Here's how the part is built. I have some questions about the finished solid (model axes, mm). A direction names the side the tool comes from. Round coordinates to 2 decimals unless told otherwise and drop trailing zeros. Loops run counter-clockwise (first coordinate to the right, second up) from the corner with the lowest first, then second, coordinate; pieces in that order, holes last. Notation, with made-up numbers: (-26.75, 74) -> (3.25, 74) arc R35 ccw to (3.25, 112) -> close; hole circle Ø10 at (76, 39). An arc over 180 degrees is marked (long way). One line per item, written item: value. Start each with the question number.
```python
from build123d import *

# Parameters (mm, degrees)
F0_W     = 4
F0_H     = 4.5
F0_W_2   = 16
F0_W_3   = 6.5
F1_DEPTH = 0.4
F2_W     = 6.5
F2_H     = 4.5
F3_DEPTH = 10


with BuildPart() as f1:
    # F0 (on Top) → F1 (new body)
    with BuildSketch(Plane.XY):
        with BuildLine():
            Line((15.75, 4.75), (15.75, 8.25))
            ThreePointArc((15.75, 8.25), (13.5533008589, 13.5533008589), (8.25, 15.75))
            Line((8.25, 15.75), (-8.25, 15.75))
            ThreePointArc((-8.25, 15.75), (-13.5533008589, 13.5533008589), (-15.75, 8.25))
            Line((-15.75, 8.25), (-15.75, -8.25))
            ThreePointArc((-15.75, -8.25), (-13.5533008589, -13.5533008589), (-8.25, -15.75))
            Line((-8.25, -15.75), (8.25, -15.75))
            ThreePointArc((8.25, -15.75), (13.5533008589, -13.5533008589), (15.75, -8.25))
            Line((15.75, -8.25), (15.75, -4.75))
            Line((15.75, -4.75), (27.3219212057, -4.75))
            ThreePointArc((27.3219212057, -4.75), (32.5853423404, -7.9993666334), (37.75, -4.5952078799))
            ThreePointArc((37.75, -4.5952078799), (42.9146576596, -7.9993666334), (48.1780787943, -4.75))
            Line((48.1780787943, -4.75), (63.9480829801, -4.75))
            ThreePointArc((63.9480829801, -4.75), (69.6474451199, -16.1274567319), (77.3637435709, -6.0087617221))
            Line((77.3637435709, -6.0087617221), (81.5596501878, 1.2587617221))
            ThreePointArc((81.5596501878, 1.2587617221), (83.4749132345, 15.4773568118), (73.9480829801, 4.75))
            Line((73.9480829801, 4.75), (48.1780787943, 4.75))
            ThreePointArc((48.1780787943, 4.75), (42.9146576596, 7.9993666334), (37.75, 4.5952078799))
            ThreePointArc((37.75, 4.5952078799), (32.5853423404, 7.9993666334), (27.3219212057, 4.75))
            Line((27.3219212057, 4.75), (15.75, 4.75))
        make_face()
        with BuildLine():
            Line((4.5, 13.25), (8.25, 13.25))
            ThreePointArc((8.25, 13.25), (11.7855339059, 11.7855339059), (13.25, 8.25))
            Line((13.25, 8.25), (13.25, 4.5))
            Line((13.25, 4.5), (13.25, 2.25))
            Line((13.25, 2.25), (29.25, 2.25))
            ThreePointArc((29.25, 2.25), (32.5, 5.5), (35.75, 2.25))
            Line((35.75, 2.25), (39.75, 2.25))
            ThreePointArc((39.75, 2.25), (43, 5.5), (46.25, 2.25))
            Line((46.25, 2.25), (74.0490381057, 2.25))
            Line((74.0490381057, 2.25), (76.1669476654, 5.9183269633))
            ThreePointArc((76.1669476654, 5.9183269633), (82.8480762114, 12.9903810568), (80.0640619824, 3.6683269633))
            Line((80.0640619824, 3.6683269633), (74.5292047573, -5.9183269633))
            ThreePointArc((74.5292047573, -5.9183269633), (67.8480762114, -12.9903810568), (70.6320904403, -3.6683269633))
            Line((70.6320904403, -3.6683269633), (71.4509618943, -2.25))
            Line((71.4509618943, -2.25), (46.25, -2.25))
            ThreePointArc((46.25, -2.25), (43, -5.5), (39.75, -2.25))
            Line((39.75, -2.25), (35.75, -2.25))
            ThreePointArc((35.75, -2.25), (32.5, -5.5), (29.25, -2.25))
            Line((29.25, -2.25), (13.25, -2.25))
            Line((13.25, -2.25), (13.25, -4.5))
            Line((13.25, -4.5), (13.25, -8.25))
            ThreePointArc((13.25, -8.25), (11.7855339059, -11.7855339059), (8.25, -13.25))
            Line((8.25, -13.25), (4.5, -13.25))
            Line((4.5, -13.25), (-4.5, -13.25))
            Line((-4.5, -13.25), (-8.25, -13.25))
            ThreePointArc((-8.25, -13.25), (-11.7855339059, -11.7855339059), (-13.25, -8.25))
            Line((-13.25, -8.25), (-13.25, -4.5))
            Line((-13.25, -4.5), (-13.25, 4.5))
            Line((-13.25, 4.5), (-13.25, 8.25))
            ThreePointArc((-13.25, 8.25), (-11.7855339059, 11.7855339059), (-8.25, 13.25))
            Line((-8.25, 13.25), (-4.5, 13.25))
            Line((-4.5, 13.25), (4.5, 13.25))
        make_face(mode=Mode.SUBTRACT)
        with Locations((37.75, 0)):
            Rectangle(F0_W, F0_H)
        with BuildLine():
            Line((4.5, 0), (4.5, 4.5))
            Line((4.5, 4.5), (0, 4.5))
            ThreePointArc((0, 4.5), (3.1819805153, 3.1819805153), (4.5, 0))
        make_face()
        with Locations((21.25, 0)):
            Rectangle(F0_W_2, F0_H)
        Polygon((74.0490381057, 2.25), (46.25, 2.25), (46.25, -2.25), (71.4509618943, -2.25), align=None)
        with BuildLine():
            ThreePointArc((13.25, 8.25), (11.7855339059, 11.7855339059), (8.25, 13.25))
            Line((8.25, 13.25), (4.5, 13.25))
            Line((4.5, 13.25), (4.5, 4.5))
            Line((4.5, 4.5), (13.25, 4.5))
            Line((13.25, 4.5), (13.25, 8.25))
        make_face()
        Polygon((4.5, 4.5), (4.5, 13.25), (-4.5, 13.25), (-4.5, 4.5), (0, 4.5), align=None)
        with BuildLine():
            Line((0, 4.5), (-4.5, 4.5))
            Line((-4.5, 4.5), (-4.5, 0))
            ThreePointArc((-4.5, 0), (-3.1819805153, 3.1819805153), (0, 4.5))
        make_face()
        with BuildLine():
            Line((-4.5, 4.5), (-4.5, 13.25))
            Line((-4.5, 13.25), (-8.25, 13.25))
            ThreePointArc((-8.25, 13.25), (-11.7855339059, 11.7855339059), (-13.25, 8.25))
            Line((-13.25, 8.25), (-13.25, 4.5))
            Line((-13.25, 4.5), (-4.5, 4.5))
        make_face()
        with BuildLine():
            ThreePointArc((0, -4.5), (-3.1819805153, -3.1819805153), (-4.5, 0))
            Line((-4.5, 0), (-4.5, -4.5))
            Line((-4.5, -4.5), (0, -4.5))
        make_face()
        Polygon((-4.5, 0), (-4.5, 4.5), (-13.25, 4.5), (-13.25, -4.5), (-4.5, -4.5), align=None)
        with BuildLine():
            Line((76.1669476654, 5.9183269633), (74.0490381057, 2.25))
            Line((74.0490381057, 2.25), (71.4509618943, -2.25))
            Line((71.4509618943, -2.25), (70.6320904403, -3.6683269633))
            ThreePointArc((70.6320904403, -3.6683269633), (72.8480762114, -4.3301270189), (74.5292047573, -5.9183269633))
            Line((74.5292047573, -5.9183269633), (80.0640619824, 3.6683269633))
            ThreePointArc((80.0640619824, 3.6683269633), (77.8480762114, 4.3301270189), (76.1669476654, 5.9183269633))
        make_face()
        with BuildLine():
            Line((13.25, -4.5), (4.5, -4.5))
            Line((4.5, -4.5), (4.5, -13.25))
            Line((4.5, -13.25), (8.25, -13.25))
            ThreePointArc((8.25, -13.25), (11.7855339059, -11.7855339059), (13.25, -8.25))
            Line((13.25, -8.25), (13.25, -4.5))
        make_face()
        Polygon((4.5, -4.5), (0, -4.5), (-4.5, -4.5), (-4.5, -13.25), (4.5, -13.25), align=None)
        with BuildLine():
            Line((-4.5, -13.25), (-4.5, -4.5))
            Line((-4.5, -4.5), (-13.25, -4.5))
            Line((-13.25, -4.5), (-13.25, -8.25))
            ThreePointArc((-13.25, -8.25), (-11.7855339059, -11.7855339059), (-8.25, -13.25))
            Line((-8.25, -13.25), (-4.5, -13.25))
        make_face()
        with BuildLine():
            ThreePointArc((0, -4.5), (3.1819805153, -3.1819805153), (4.5, 0))
            ThreePointArc((4.5, 0), (3.1819805153, 3.1819805153), (0, 4.5))
            ThreePointArc((0, 4.5), (-3.1819805153, 3.1819805153), (-4.5, 0))
            ThreePointArc((-4.5, 0), (-3.1819805153, -3.1819805153), (0, -4.5))
        make_face()
        with BuildLine():
            ThreePointArc((35.75, 2.25), (32.5, 5.5), (29.25, 2.25))
            Line((29.25, 2.25), (35.75, 2.25))
        make_face()
        with BuildLine():
            Line((4.5, -4.5), (4.5, 0))
            ThreePointArc((4.5, 0), (3.1819805153, -3.1819805153), (0, -4.5))
            Line((0, -4.5), (4.5, -4.5))
        make_face()
        with BuildLine():
            Line((46.25, -2.25), (39.75, -2.25))
            ThreePointArc((39.75, -2.25), (43, -5.5), (46.25, -2.25))
        make_face()
        with BuildLine():
            ThreePointArc((46.25, 2.25), (43, 5.5), (39.75, 2.25))
            Line((39.75, 2.25), (46.25, 2.25))
        make_face()
        with BuildLine():
            Line((35.75, -2.25), (29.25, -2.25))
            ThreePointArc((29.25, -2.25), (32.5, -5.5), (35.75, -2.25))
        make_face()
        with BuildLine():
            ThreePointArc((74.5292047573, -5.9183269633), (72.8480762114, -4.3301270189), (70.6320904403, -3.6683269633))
            ThreePointArc((70.6320904403, -3.6683269633), (67.8480762114, -12.9903810568), (74.5292047573, -5.9183269633))
        make_face()
        with BuildLine():
            ThreePointArc((80.0640619824, 3.6683269633), (82.8480762114, 12.9903810568), (76.1669476654, 5.9183269633))
            ThreePointArc((76.1669476654, 5.9183269633), (77.8480762114, 4.3301270189), (80.0640619824, 3.6683269633))
        make_face()
        Polygon((13.25, 4.5), (4.5, 4.5), (4.5, 0), (4.5, -4.5), (13.25, -4.5), (13.25, -2.25), (13.25, 2.25), align=None)
        with Locations((32.5, 0)):
            Rectangle(F0_W_3, F0_H)
        with Locations((43, 0)):
            Rectangle(F0_W_3, F0_H)
    extrude(amount=F1_DEPTH)

    # F2 (on face) → F3 (join)
    with BuildSketch(Plane.XY.offset(0.4)):
        with BuildLine():
            Line((4.5, -4.5), (4.5, 0))
            ThreePointArc((4.5, 0), (3.1819805153, -3.1819805153), (0, -4.5))
            Line((0, -4.5), (4.5, -4.5))
        make_face()
        with BuildLine():
            ThreePointArc((0, -4.5), (3.1819805153, -3.1819805153), (4.5, 0))
            ThreePointArc((4.5, 0), (3.1819805153, 3.1819805153), (0, 4.5))
            ThreePointArc((0, 4.5), (-3.1819805153, 3.1819805153), (-4.5, 0))
            ThreePointArc((-4.5, 0), (-3.1819805153, -3.1819805153), (0, -4.5))
        make_face()
        with BuildLine():
            Line((4.5, 0), (4.5, 4.5))
            Line((4.5, 4.5), (0, 4.5))
            ThreePointArc((0, 4.5), (3.1819805153, 3.1819805153), (4.5, 0))
        make_face()
        with BuildLine():
            Line((0, 4.5), (-4.5, 4.5))
            Line((-4.5, 4.5), (-4.5, 0))
            ThreePointArc((-4.5, 0), (-3.1819805153, 3.1819805153), (0, 4.5))
        make_face()
        with BuildLine():
            ThreePointArc((0, -4.5), (-3.1819805153, -3.1819805153), (-4.5, 0))
            Line((-4.5, 0), (-4.5, -4.5))
            Line((-4.5, -4.5), (0, -4.5))
        make_face()
        Polygon((13.25, 4.5), (4.5, 4.5), (4.5, 0), (4.5, -4.5), (13.25, -4.5), (13.25, -2.25), (13.25, 2.25), align=None)
        with BuildLine():
            Line((-4.5, 4.5), (-4.5, 13.25))
            Line((-4.5, 13.25), (-8.25, 13.25))
            ThreePointArc((-8.25, 13.25), (-11.7855339059, 11.7855339059), (-13.25, 8.25))
            Line((-13.25, 8.25), (-13.25, 4.5))
            Line((-13.25, 4.5), (-4.5, 4.5))
        make_face()
        Polygon((-4.5, 0), (-4.5, 4.5), (-13.25, 4.5), (-13.25, -4.5), (-4.5, -4.5), align=None)
        with BuildLine():
            ThreePointArc((13.25, 8.25), (11.7855339059, 11.7855339059), (8.25, 13.25))
            Line((8.25, 13.25), (4.5, 13.25))
            Line((4.5, 13.25), (4.5, 4.5))
            Line((4.5, 4.5), (13.25, 4.5))
            Line((13.25, 4.5), (13.25, 8.25))
        make_face()
        Polygon((4.5, 4.5), (4.5, 13.25), (-4.5, 13.25), (-4.5, 4.5), (0, 4.5), align=None)
        Polygon((4.5, -4.5), (0, -4.5), (-4.5, -4.5), (-4.5, -13.25), (4.5, -13.25), align=None)
        with BuildLine():
            Line((-4.5, -13.25), (-4.5, -4.5))
            Line((-4.5, -4.5), (-13.25, -4.5))
            Line((-13.25, -4.5), (-13.25, -8.25))
            ThreePointArc((-13.25, -8.25), (-11.7855339059, -11.7855339059), (-8.25, -13.25))
            Line((-8.25, -13.25), (-4.5, -13.25))
        make_face()
        with BuildLine():
            Line((13.25, -4.5), (4.5, -4.5))
            Line((4.5, -4.5), (4.5, -13.25))
            Line((4.5, -13.25), (8.25, -13.25))
            ThreePointArc((8.25, -13.25), (11.7855339059, -11.7855339059), (13.25, -8.25))
            Line((13.25, -8.25), (13.25, -4.5))
        make_face()
        with Locations((32.5, 0)):
            Rectangle(F2_W, F2_H)
        with BuildLine():
            ThreePointArc((35.75, 2.25), (32.5, 5.5), (29.25, 2.25))
            Line((29.25, 2.25), (35.75, 2.25))
        make_face()
        with BuildLine():
            Line((35.75, -2.25), (29.25, -2.25))
            ThreePointArc((29.25, -2.25), (32.5, -5.5), (35.75, -2.25))
        make_face()
        with BuildLine():
            Line((46.25, -2.25), (39.75, -2.25))
            ThreePointArc((39.75, -2.25), (43, -5.5), (46.25, -2.25))
        make_face()
        with Locations((43, 0)):
            Rectangle(F2_W, F2_H)
        with BuildLine():
            ThreePointArc((46.25, 2.25), (43, 5.5), (39.75, 2.25))
            Line((39.75, 2.25), (46.25, 2.25))
        make_face()
        with BuildLine():
            ThreePointArc((72.8480762114, -4.3301270189), (71.7788727151, -3.8693437522), (70.6320904403, -3.6683269633))
            ThreePointArc((70.6320904403, -3.6683269633), (67.8480762114, -12.9903810568), (74.5292047573, -5.9183269633))
            ThreePointArc((74.5292047573, -5.9183269633), (73.7817279741, -5.0256927751), (72.8480762114, -4.3301270189))
        make_face()
        with BuildLine():
            ThreePointArc((80.0640619824, 3.6683269633), (82.8480762114, 12.9903810568), (76.1669476654, 5.9183269633))
            ThreePointArc((76.1669476654, 5.9183269633), (76.9144244486, 5.0256927751), (77.8480762114, 4.3301270189))
            ThreePointArc((77.8480762114, 4.3301270189), (78.9172797076, 3.8693437522), (80.0640619824, 3.6683269633))
        make_face()
    extrude(amount=F3_DEPTH)


solid = f1.part
```
Q1. I want a section at D-D on x = 25. Please give me the cut outline in (y, z), plus the area to 3 significant figures.
Q2. Will these pins go through, and if not, where does the flat tip stop? P1, Ø6, axis at y = 11, z = 7.5, coming from the +X side; P2, Ø4, axis at x = 61, z = 1, coming from the +Y side; P3, Ø3.5, axis at y = 1, z = 7, coming from the +X side.
Q3. If we mould it in two halves opening along X, with no side actions, what happens to faces 6 (the cylindrical face through (-13.611, -13.495, 0.197)), 7 (the cylindrical face through (32.5, -8, 0.2)), 8 (the flat face through (0, 13.25, 5))? For each: released by +X, released by -X, zero draft, split by the parting line, or undercut.
Q4. If I drill on line 1 along X through (y, z) = (-3.5, 4); line 2 along X through (y, z) = (2.5, 9.5); line 3 along X through (y, z) = (8.5, 9), over which ranges is the centre line in solid material (lowest first)?
Q5. I want a section at B-B on x = 0. Please give me the cut outline in (y, z), plus the area to 3 significant figures.
Q6. I want a section at C-C on x = 43. Please give me the cut outline in (y, z), plus the area to 3 significant figures.
Q7. Which directions (+Z, -Z, +X, -X, +Y, -Y) give clear straight access to the entire face, cutting with the end or side of a thin tool? Please do faces 1 (the cylindrical face through (13.495, -13.611, 0.197)), 2 (the cylindrical face through (43.1, 5.5, 5.3)), 3 (the flat face through (13.25, 0, 5)), 4 (the flat face through (39.6, 2.5, 0.4)), 5 (the cylindrical face through (42.9, -5.5, 5.3)).
Q8. I want a section at A-A on z = 9.5. Please give me the cut outline in (x, y).
Answers below:
1. outline: (-4.75, 0) -> (4.75, 0) -> (4.75, 0.4) -> (-4.75, 0.4) -> close
1. area: 3.80 mm^2
2. P1: stops at x = 85.35
2. P2: stops at y = 4.75
2. P3: stops at x = 46.25
3. face 6: released by -X
3. face 7: undercut
3. face 8: zero draft
4. line 1: x = -13.25 to 13.25, 29.5 to 35.5, 40 to 46
4. line 2: x = -13.25 to 13.25, 29.26 to 35.74, 39.76 to 46.24
4. line 3: x = -13.24 to 13.24, 75.35 to 85.35
5. outline: (-15.75, 0) -> (15.75, 0) -> (15.75, 0.4) -> (13.25, 0.4) -> (13.25, 10.4) -> (-13.25, 10.4) -> (-13.25, 0.4) -> (-15.75, 0.4) -> close
5. area: 278 mm^2
6. outline: (-8, 0) -> (8, 0) -> (8, 0.4) -> (5.5, 0.4) -> (5.5, 10.4) -> (-5.5, 10.4) -> (-5.5, 0.4) -> (-8, 0.4) -> close
6. area: 116 mm^2
7. face 1: +Z, -Z, -Y
7. face 2: +Z, +Y
7. face 3: +Z, +Y, -Y
7. face 4: +Z
7. face 5: +Z, -Y
8. outline: (-13.25, -8.25) arc R5 ccw to (-8.25, -13.25) -> (8.25, -13.25) arc R5 ccw to (13.25, -8.25) -> (13.25, 8.25) arc R5 ccw to (8.25, 13.25) -> (-8.25, 13.25) arc R5 ccw to (-13.25, 8.25) -> close; (29.25, -2.25) arc R3.25 ccw to (35.75, -2.25) -> (35.75, 2.25) arc R3.25 ccw to (29.25, 2.25) -> close; (39.75, -2.25) arc R3.25 ccw to (46.25, -2.25) -> (46.25, 2.25) arc R3.25 ccw to (39.75, 2.25) -> close; circle Ø10 at (70.35, -8.66); circle Ø10 at (80.35, 8.66)
